Work out the finished part from the listing and answer in its coordinate system (mm). Face numbers are marked on the shaded views. Give positions to 0.01 mm unless a question says otherwise; leave off trailing zeros. Loops run counter-clockwise (first coordinate to the right, second up) from the corner with the lowest first, then second, coordinate; pieces in that order, holes last. Notation, with made-up numbers: (-12.5, -23) - (8.5, -23) arc R26 ccw to (8.5, 0) - close; hole circle Ø2 at (-25.5, 22). An arc over 180 degrees is marked (long way). One line per question, with ' | ' between items. Start each with the question number.
1. For a pull along X with two mould halves and no side action, classify the marked faces 1, 2 and 3 as released by +X, released by -X, zero draft, split by the parting line, or undercut.
2. Each of these flat-tipped pins is pushed along its axis until it touches: pin 1 (0.5 mm diameter, centred on x = 12, y = -10, fed in from +Z); pin 2 (22 mm diameter, centred on x = 5, y = 7, fed in from -Z); pin 3 (4.5 mm diameter, centred on x = 17, y = 8.5, fed in from +Z); pin 4 (6 mm diameter, centred on x = 9, z = 17, fed in from -Y). Where does it stop, or does it pass through?
3. Find the intervals of material crossed by line 1 (X direction, y = -18, z = 1.5); line 2 (X direction, y = 0, z = 14.75); line 3 (Y direction, x = 5, z = 6), in increasing order.
4. Section B-B (x = 28) is taken. Determine the outline of the cut face in (y, z).
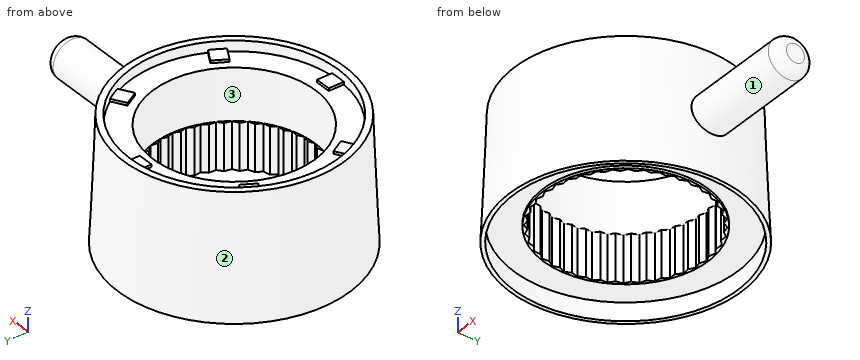
from build123d import *

# Parameters (mm, degrees)
F0_R           = 22.5
F2_R           = 21.5
F4_R           = 20.25
F5_DEPTH       = 2
F6_R           = 21.75
F7_DEPTH       = 3.5
F8_R           = 15.75
F9_DEPTH       = 18.5
F10_W          = 3
F10_H          = 3
F11_DEPTH      = 0.5
F14_R          = 16
F15_DEPTH      = 8.5
F15_DEPTH_BACK = 0.5
F18_R          = 3.75
F19_DEPTH      = 23
F20_R          = 2


with BuildPart() as f3:
    # F0 (on Top) → F3 section 0
    with BuildSketch(Plane.XY):
        Circle(F0_R)
    # F2 (on offset) → F3 section 1
    with BuildSketch(Plane.XY.offset(24)):
        Circle(F2_R)
    loft()

    # F4 (on face) → F5 (cut)
    with BuildSketch(Plane.XY.offset(24)):
        Circle(F4_R)
    extrude(amount=-F5_DEPTH, mode=Mode.SUBTRACT)

    # F6 (on face) → F7 (cut)
    with BuildSketch(Plane(origin=(0, 0, 0), x_dir=(1, 0, 0), z_dir=(0, 0, -1))):
        Circle(F6_R)
    extrude(amount=-F7_DEPTH, mode=Mode.SUBTRACT)

    # F8 (on face) → F9 (cut, through all)
    with BuildSketch(Plane.XY.offset(22)):
        Circle(F8_R)
    extrude(amount=-F9_DEPTH, mode=Mode.SUBTRACT)

    # F10 (on face) → F11 (join)
    with BuildSketch(Plane.XY.offset(22)):
        with Locations((0, 18.75)):
            Rectangle(F10_W, F10_H)
        Polygon((-15.6889382153, 7.3259618943), (-14.1889382153, 9.9240381057), (-16.7870144266, 11.4240381057), (-18.2870144266, 8.8259618943), align=None)
        Polygon((-14.1889382153, -9.9240381057), (-15.6889382153, -7.3259618943), (-18.2870144266, -8.8259618943), (-16.7870144266, -11.4240381057), align=None)
        with Locations((0, -18.75)):
            Rectangle(F10_W, F10_H)
        Polygon((15.6889382153, -7.3259618943), (14.1889382153, -9.9240381057), (16.7870144266, -11.4240381057), (18.2870144266, -8.8259618943), align=None)
        Polygon((14.1889382153, 9.9240381057), (15.6889382153, 7.3259618943), (18.2870144266, 8.8259618943), (16.7870144266, 11.4240381057), align=None)
    extrude(amount=F11_DEPTH)

    # F14 (on face) → F15 (join, two sides)
    with BuildSketch(Plane(origin=(0, 0, 3.5), x_dir=(1, 0, 0), z_dir=(0, 0, -1))) as f15_sk:
        Circle(F14_R)
        Polygon((-1.1965012098, 15.2029893394), (0, 15.75), (1.1965012098, 15.2029893394), (2.4638428244, 15.5560913644), (3.5600417988, 14.8286412861), (4.8670176614, 14.9791401316), (5.8359223436, 14.0891628708), (7.1503503709, 14.033352756), (7.9681031119, 13.0027625064), (9.2576177236, 12.7420176614), (9.904082737, 11.5961909754), (11.1369318037, 11.1369318037), (11.5961909754, 9.904082737), (12.7420176614, 9.2576177236), (13.0027625064, 7.9681031119), (14.033352756, 7.1503503709), (14.0891628708, 5.8359223436), (14.9791401316, 4.8670176614), (14.8286412861, 3.5600417988), (15.5560913644, 2.4638428244), (15.2029893394, 1.1965012098), (15.75, 0), (15.2029893394, -1.1965012098), (15.5560913644, -2.4638428244), (14.8286412861, -3.5600417988), (14.9791401316, -4.8670176614), (14.0891628708, -5.8359223436), (14.033352756, -7.1503503709), (13.0027625064, -7.9681031119), (12.7420176614, -9.2576177236), (11.5961909754, -9.904082737), (11.1369318037, -11.1369318037), (9.904082737, -11.5961909754), (9.2576177236, -12.7420176614), (7.9681031119, -13.0027625064), (7.1503503709, -14.033352756), (5.8359223436, -14.0891628708), (4.8670176614, -14.9791401316), (3.5600417988, -14.8286412861), (2.4638428244, -15.5560913644), (1.1965012098, -15.2029893394), (0, -15.75), (-1.1965012098, -15.2029893394), (-2.4638428244, -15.5560913644), (-3.5600417988, -14.8286412861), (-4.8670176614, -14.9791401316), (-5.8359223436, -14.0891628708), (-7.1503503709, -14.033352756), (-7.9681031119, -13.0027625064), (-9.2576177236, -12.7420176614), (-9.904082737, -11.5961909754), (-11.1369318037, -11.1369318037), (-11.5961909754, -9.904082737), (-12.7420176614, -9.2576177236), (-13.0027625064, -7.9681031119), (-14.033352756, -7.1503503709), (-14.0891628708, -5.8359223436), (-14.9791401316, -4.8670176614), (-14.8286412861, -3.5600417988), (-15.5560913644, -2.4638428244), (-15.2029893394, -1.1965012098), (-15.75, 0), (-15.2029893394, 1.1965012098), (-15.5560913644, 2.4638428244), (-14.8286412861, 3.5600417988), (-14.9791401316, 4.8670176614), (-14.0891628708, 5.8359223436), (-14.033352756, 7.1503503709), (-13.0027625064, 7.9681031119), (-12.7420176614, 9.2576177236), (-11.5961909754, 9.904082737), (-11.1369318037, 11.1369318037), (-9.904082737, 11.5961909754), (-9.2576177236, 12.7420176614), (-7.9681031119, 13.0027625064), (-7.1503503709, 14.033352756), (-5.8359223436, 14.0891628708), (-4.8670176614, 14.9791401316), (-3.5600417988, 14.8286412861), (-2.4638428244, 15.5560913644), align=None, mode=Mode.SUBTRACT)
    extrude(amount=-F15_DEPTH)
    extrude(f15_sk.sketch, amount=F15_DEPTH_BACK)

    # F18 (on offset) → F19 (join)
    with BuildSketch(Plane.YZ.offset(20.25)):
        with Locations((0, 12)):
            Circle(F18_R)
    extrude(amount=F19_DEPTH)

    # F20
    f20_edges = [f3.edges().sort_by_distance(p)[0] for p in [
        (43.25, -3.75, 12),
    ]]
    fillet(f20_edges, radius=F20_R)


solid = f3.part
Conclusion:
1) face 1: zero draft | face 2: split by the parting line | face 3: undercut
2) pin 1: z = 22 | pin 2: z = 3 | pin 3: z = 24 | pin 4: y = -20.96
3) line 1: -13.4 to -12.21, 12.21 to 13.4 | line 2: -21.89 to -15.75, 15.75 to 42.98 | line 3: -21.68 to -14.86, 14.86 to 21.68
4) outline: circle Ø7.5 at (0, 12)
